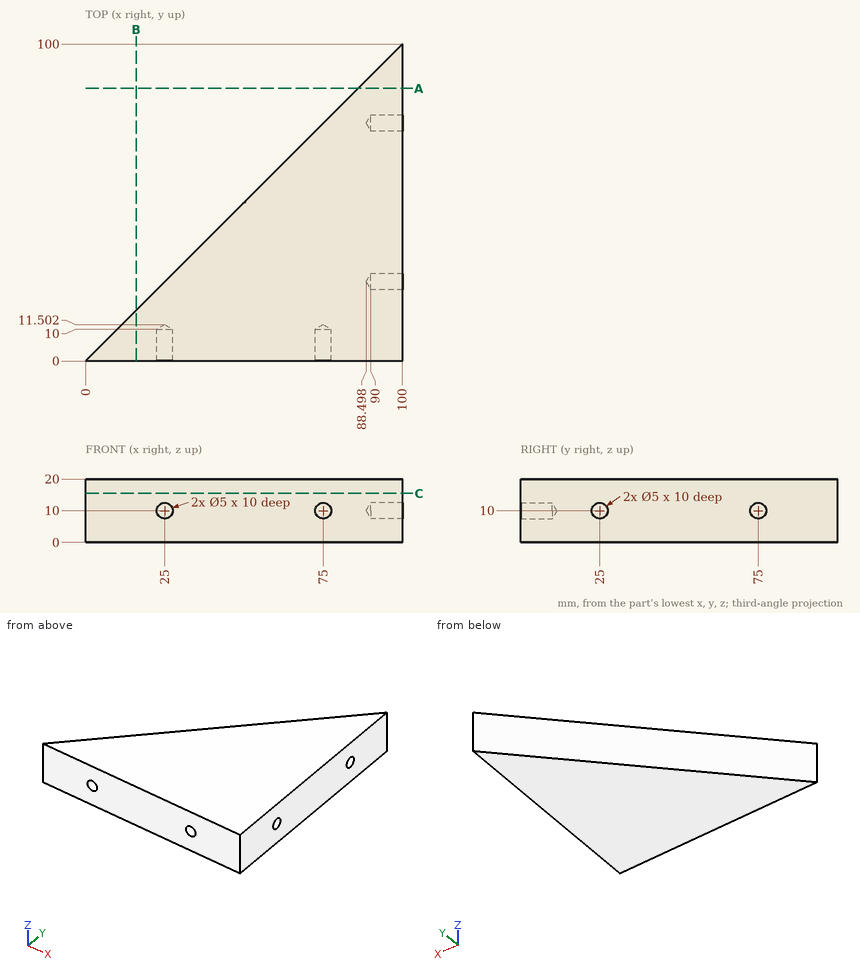
Answer from the drawing. Dimensions are ordinates in mm from the lowest x, y and z of the part. Coordinates: 2 decimals unless noted, no trailing zeros. Loops run counter-clockwise (first coordinate to the right, second up) from the corner with the lowest first, then second, coordinate; pieces in that order, holes last.
Q1. Consider probe 1 along X at (y, z) = (7.5, 10); probe 2 along Z at (x, y) = (95, 25); probe 3 along Y at (x, z) = (92.5, 10). Determine where each line is inside the solid, lowest interval first.
Q2. Each of these flat-tipped pins is pushed along its axis until it touches: pin 1 Ø2 at (y, z) = (84.5, 3) entering from -X; pin 2 Ø1 at (y, z) = (33.5, 7.5) entering from -X; pin 3 Ø8 at (y, z) = (25, 10) entering from +X; pin 4 Ø5 at (y, z) = (63.5, 8) entering from -X. Where does it stop, or does it pass through?
Q3. The part is cut by section A-A on y = 86. Write down the section's boundary in (x, z), and give its area (3 significant figures).
Q4. The part is cut by section C-C on z = 15.5. Write down the section's boundary in (x, y).
Q5. The part is cut by section B-B on x = 16. Write down the section's boundary in (y, z), and give its area (3 significant figures).
Results below:
1. probe 1: x = 7.5 to 22.5, 27.5 to 72.5, 77.5 to 100
1. probe 2: z = 0 to 7.5, 12.5 to 20
1. probe 3: y = 0 to 22.5, 27.5 to 72.5, 77.5 to 92.5
2. pin 1: stops at x = 83.5
2. pin 2: stops at x = 33
2. pin 3: stops at x = 100
2. pin 4: stops at x = 61
3. outline: (86, 0) - (100, 0) - (100, 20) - (86, 20) - close
3. area: 280 mm2
4. outline: (0, 0) - (100, 0) - (100, 100) - close
5. outline: (0, 0) - (16, 0) - (16, 20) - (0, 20) - close
5. area: 320 mm2
